Read the model definition and answer for the solid it produces. Units are mm, in the model's axes. A direction names the side the tool comes from. Give positions to 0.01 mm unless a question says otherwise; leave off trailing zeros. Write each loop counter-clockwise with the first axis right and the second up, starting at its lowest first coordinate (ties: lowest second). Pieces come first, ordered by that corner, then holes. Notation, with made-up numbers: M 36,-36 L 51,-36 A18 ccw 51,-13 Z; hole C 70.25,-39.5 d6. An arc over 180 degrees is marked long. Use a Markdown table: item, result. Add a question column.
Item 1: Consider probe 1 along Y at (x, z) = (89.21, 2.65); probe 2 along Y at (x, z) = (121, 6); probe 3 along Z at (x, y) = (118, -42.5). Determine where each line is inside the solid, lowest interval first. Write a range as [from, to].
Item 2: The mould has two halves that part along X. Classify faces 6 (the flat face through (13.665, -32, 6)), 7 (the flat face through (121.768, -32, 6)), 8 (the flat face through (86, -48.26, 6)), 9 (the flat face through (25.044, -32, 6)): pulls with the +X half, pulls with the -X half, needs draft (parallel to the pull), parting line crosses it, or undercut.
Item 3: A cutting plane is placed at C-C on z = 6. Count the separate pieces of the cut face and the enclosed holes in it, then the cut area to 3 significant figures.
Item 4: Given P1, Ø1.8, axis at x = 69.5, z = 6, coming from the +Y side; P2, Ø2, axis at y = -29, z = 6.5, coming from the +X side; P3, Ø0.7, axis at x = 36, z = 5.5, coming from the -Y side, each flat-ended and moving along its own axis, determine where each tip first touches the part or whether it passes through.
Item 5: For faces 1 (the flat face through (63, 0, 2)), 2 (the flat face through (30, -32, 7.099)), 3 (the flat face through (13, -16.256, 6)), 4 (the flat face through (19.355, -32, 6)), 5 (the flat face through (18, -48.26, 6)), determine the directions among +Z, -Z, +X, -X, +Y, -Y from which every point of the face is accessible in a straight line to the end or side of a thin tool.
Item 6: A cutting plane is placed at A-A on x = 89.21. Determine the outline of the cut face in (y, z).
Item 7: A cutting plane is placed at B-B on x = 58. Determine the outline of the cut face in (y, z), then the cut area to 3 significant figures.
from build123d import *

# Parameters (mm, degrees)
F0_W     = 127.07
F0_H     = 50.8
F0_R     = 2.5
F1_DEPTH = 4.3053
F2_W     = 2.286
F2_H     = 32.004
F3_DEPTH = 2.794


with BuildPart() as f1:
    # F0 (on Top) → F1 (new body)
    with BuildSketch(Plane.XY):
        with Locations((63.535, -25.4)):
            Rectangle(F0_W, F0_H)
        with Locations((38.2335, -9.144)):
            Circle(F0_R, mode=Mode.SUBTRACT)
        with Locations((89.21, -9.144)):
            Circle(F0_R, mode=Mode.SUBTRACT)
    extrude(amount=F1_DEPTH)

    # F2 (on face) → F3 (join)
    with BuildSketch(Plane.XY.offset(4.3053)):
        with Locations((1.143, -32.258)):
            Rectangle(F2_W, F2_H)
        with Locations((6.8326, -32.258)):
            Rectangle(F2_W, F2_H)
        with Locations((12.5222, -32.258)):
            Rectangle(F2_W, F2_H)
        with Locations((18.2118, -32.258)):
            Rectangle(F2_W, F2_H)
        with Locations((23.9014, -32.258)):
            Rectangle(F2_W, F2_H)
        with Locations((29.591, -32.258)):
            Rectangle(F2_W, F2_H)
        with Locations((35.2806, -32.258)):
            Rectangle(F2_W, F2_H)
        with Locations((40.9702, -32.258)):
            Rectangle(F2_W, F2_H)
        with Locations((46.6598, -32.258)):
            Rectangle(F2_W, F2_H)
        with Locations((52.3494, -32.258)):
            Rectangle(F2_W, F2_H)
        with Locations((58.039, -32.258)):
            Rectangle(F2_W, F2_H)
        with Locations((63.7286, -32.258)):
            Rectangle(F2_W, F2_H)
        with Locations((69.4182, -32.258)):
            Rectangle(F2_W, F2_H)
        with Locations((75.1078, -32.258)):
            Rectangle(F2_W, F2_H)
        with Locations((80.7974, -32.258)):
            Rectangle(F2_W, F2_H)
        with Locations((86.487, -32.258)):
            Rectangle(F2_W, F2_H)
        with Locations((92.1766, -32.258)):
            Rectangle(F2_W, F2_H)
        with Locations((97.8662, -32.258)):
            Rectangle(F2_W, F2_H)
        with Locations((103.5558, -32.258)):
            Rectangle(F2_W, F2_H)
        with Locations((109.2454, -32.258)):
            Rectangle(F2_W, F2_H)
        with Locations((114.935, -32.258)):
            Rectangle(F2_W, F2_H)
        with Locations((120.6246, -32.258)):
            Rectangle(F2_W, F2_H)
    extrude(amount=F3_DEPTH)


solid = f1.part
Filled in:
| question | item | result |
|---|---|---|
| 1 | probe 1 | [-50.8, -11.64], [-6.64, 0] |
| 1 | probe 2 | [-48.26, -16.26] |
| 1 | probe 3 | [0, 4.31] |
| 2 | face 6 | undercut |
| 2 | face 7 | pulls with the +X half |
| 2 | face 8 | needs draft |
| 2 | face 9 | undercut |
| 3 | separate pieces | 22 |
| 3 | enclosed holes | 0 |
| 3 | area | 1,610 mm² |
| 4 | P1 | y = -16.26 |
| 4 | P2 | x = 121.77 |
| 4 | P3 | y = -48.26 |
| 5 | face 1 | +Z, -Z, +X, -X, +Y |
| 5 | face 2 | +Z, +X, -X, +Y, -Y |
| 5 | face 3 | +Z, +X, -X, +Y |
| 5 | face 4 | +Z, +Y, -Y |
| 5 | face 5 | +Z, +X, -X, -Y |
| 6 | outline | M -50.8,0 L -11.64,0 L -11.64,4.31 L -50.8,4.31 Z; M -6.64,0 L 0,0 L 0,4.31 L -6.64,4.31 Z |
| 7 | outline | M -50.8,0 L 0,0 L 0,4.31 L -16.26,4.31 L -16.26,7.1 L -48.26,7.1 L -48.26,4.31 L -50.8,4.31 Z |
| 7 | area | 308 mm² |
